```python
from build123d import *

# Parameters (mm, degrees)
ESBO_O18_W                 = 111.5
ESBO_O18_H                 = 54.5
RESSALTO_EXTRUS_O2_DEPTH   = 1.4
ESBO_O19_W                 = 117.5
ESBO_O19_H                 = 61
RESSALTO_EXTRUS_O3_DEPTH   = 2
ESBO_O24_R                 = 1
CORTE_EXTRUS_O1_DEPTH      = 86.215413827
CORTE_EXTRUS_O3_DEPTH      = 86.460885308
CORTE_EXTRUS_O3_DEPTH_BACK = 86.460885308
ESBO_O25_R                 = 7.8
ESBO_O25_R_2               = 4.186600547
CORTE_EXTRUS_O8_DEPTH      = 86.215413827


with BuildPart() as part:
    # Esboço18 → Ressalto-extrusão2 (new body)
    with BuildSketch(Plane(origin=(0, 0, 0), x_dir=(1, 0, 0), z_dir=(0, 1, 0))):
        with Locations((20.747526714, 0)):
            Rectangle(ESBO_O18_W, ESBO_O18_H)
    extrude(amount=RESSALTO_EXTRUS_O2_DEPTH)

    # Esboço19 → Ressalto-extrusão3 (add)
    with BuildSketch(Plane(origin=(0, 1.4, 0), x_dir=(1, 0, 0), z_dir=(0, 1, 0))):
        with Locations((20.747526714, 0)):
            Rectangle(ESBO_O19_W, ESBO_O19_H)
    extrude(amount=RESSALTO_EXTRUS_O3_DEPTH)

    # Esboço24 → Corte-extrusão1 (cut, through all)
    with BuildSketch(Plane(origin=(0, 3.4, 0), x_dir=(1, 0, 0), z_dir=(0, 1, 0))):
        with Locations(Location((-36.252473286, 28.75, 0), (0, 0, 270))):
            Circle(ESBO_O24_R)
        with Locations(Location((77.747526714, 28.75, 0), (0, 0, 270))):
            Circle(ESBO_O24_R)
        with Locations(Location((77.747526714, -28.75, 0), (0, 0, 270))):
            Circle(ESBO_O24_R)
        with Locations(Location((-36.25, -28.75, 0), (0, 0, 270))):
            Circle(ESBO_O24_R)
    extrude(amount=-CORTE_EXTRUS_O1_DEPTH, mode=Mode.SUBTRACT)

    # Esboço25 → Corte-extrusão3 (cut, two sides: drawn at the far end of the back side and taken through both)
    # profile 1 of 3: a face of its own
    with BuildSketch(Plane(origin=(0, 7.31137223, 0), x_dir=(1, 0, 0), z_dir=(0, 1, 0)).offset(-CORTE_EXTRUS_O3_DEPTH_BACK)):
        with Locations(Location((-16.682939742, 11.661108672, 0), (0, 0, 180))):
            Circle(ESBO_O25_R)
        with Locations((-16.682939742, 11.661108672)):
            Circle(ESBO_O25_R_2, mode=Mode.SUBTRACT)
    # profile 2 of 3: a face of its own
    with BuildSketch(Plane(origin=(0, 7.31137223, 0), x_dir=(1, 0, 0), z_dir=(0, 1, 0)).offset(-CORTE_EXTRUS_O3_DEPTH_BACK)):
        with Locations((-16.682939742, 11.661108672)):
            Circle(ESBO_O25_R_2)
    # profile 3 of 3: a face of its own
    with BuildSketch(Plane(origin=(0, 7.31137223, 0), x_dir=(1, 0, 0), z_dir=(0, 1, 0)).offset(-CORTE_EXTRUS_O3_DEPTH_BACK)):
        with Locations(Location((-16.710330787, -11.680669769, 0), (0, 0, 180))):
            Circle(ESBO_O25_R)
    extrude(amount=CORTE_EXTRUS_O3_DEPTH + CORTE_EXTRUS_O3_DEPTH_BACK, mode=Mode.SUBTRACT)

    # Esboço26 → Corte-extrusão8 (cut, through all)
    with BuildSketch(Plane(origin=(0, 0, 0), x_dir=(1, 0, 0), z_dir=(0, 1, 0))):
        with BuildLine():
            Line((58.447526714, -11.55), (58.447526714, -21.55))
            ThreePointArc((58.447526714, -21.55), (60.947526714, -16.55), (58.447526714, -11.55))
        make_face()
        with BuildLine():
            Line((55.947526714, -10.426275643), (55.947526714, -22.673724357))
            ThreePointArc((55.947526714, -22.673724357), (54.697526714, -22.8), (53.447526714, -22.673724357))
            Line((53.447526714, -22.673724357), (53.447526714, -10.426275643))
            ThreePointArc((53.447526714, -10.426275643), (54.697526714, -10.3), (55.947526714, -10.426275643))
        make_face()
        with BuildLine():
            Line((50.947526714, -11.55), (50.947526714, -21.55))
            ThreePointArc((50.947526714, -21.55), (48.447526714, -16.55), (50.947526714, -11.55))
        make_face()
    extrude(amount=CORTE_EXTRUS_O8_DEPTH, mode=Mode.SUBTRACT)


solid = part.part
```
Model file for the job. Use its own axes, mm. A direction names the side the tool comes from. Round coordinates to 2 decimals unless told otherwise and drop trailing zeros. Write each loop counter-clockwise with the first axis right and the second up, starting at its lowest first coordinate (ties: lowest second). Pieces come first, ordered by that corner, then holes. Notation, with made-up numbers: M 69,33 L 105,33 A19 ccw 105,40 Z; hole C -14,75 d7. An arc over 180 degrees is marked long. Put each result on its own line as item: value.
Item 1: Cut at A-A (y = 2.1). State how many separate pieces and enclosed holes the cut face has, and give its area (3 significant figures).
Responses:
separate pieces: 1
enclosed holes: 9
area: 6,710 mm²
Item 2: Mould opens along Z. For faces 3 (the flat face through (20, 2, 30.5)), 4 (the cylindrical face through (-35.41, 2.41, 29.29)), 5 (the flat face through (20, 2, -30.5)), 6 (the flat face through (79.498, 2, 0)) say: +Z half, -Z half, draft (parallel to the pull), parting line (faces both ways), or undercut.
Responses:
face 3: +Z half
face 4: undercut
face 5: -Z half
face 6: draft
Item 3: Cut at B-B (z = -25). List the corners of the cut face in (x, y), and give its area (3 significant figures).
Responses:
outline: M -38,1.4 L -35,1.4 L -35,0 L 76.5,0 L 76.5,1.4 L 79.5,1.4 L 79.5,3.4 L -38,3.4 Z
area: 391 mm²
Item 4: Cut at D-D (z = -8). List the corners of the cut face in (x, y), and give its area (3 significant figures).
Responses:
outline: M -38,1.4 L -35,1.4 L -35,0 L -23.57,0 L -23.57,3.4 L -38,3.4 Z; M -9.8,0 L 76.5,0 L 76.5,1.4 L 79.5,1.4 L 79.5,3.4 L -9.8,3.4 Z
area: 344 mm²
Item 5: Flat gauge pins, fed straight in: P1, Ø1.5, axis at y = 0.5, z = -2, coming from the -X side; P2, Ø2.5, axis at x = -36.25, z = 28.75, coming from the -Y side. Where does each tip first touch, or does it go through?
Responses:
P1: x = -35
P2: y = 1.4
Item 6: Tool access for faces 1 (the flat face through (20, 0, 0)), 2 (the cylindrical face through (54.7, 1.7, 22.8)): list every direction of +Z, -Z, +X, -X, +Y, -Y with a clear straight run to the whole face (end or side of a thin tool).
Responses:
face 1: +Z, -Z, +X, -X, -Y
face 2: +Y, -Y
Item 7: Probe L1, parallel to X at y = 2.4, z = -28.75; L2, parallel to Z at x = -23.5, y = 2.45. List the from-to ranges inside material, lowest first. Write a range as from..to.
Responses:
L1: -38..-37.25, -35.25..76.75, 78.75..79.5
L2: -30.5..-15.45, -7.87..7.84, 15.52..30.5
Item 8: Cut at C-C (x = 14.5). List the corners of the cut face in (y, z).
Responses:
outline: M 0,-27.25 L 1.4,-27.25 L 1.4,-30.5 L 3.4,-30.5 L 3.4,30.5 L 1.4,30.5 L 1.4,27.25 L 0,27.25 Z
